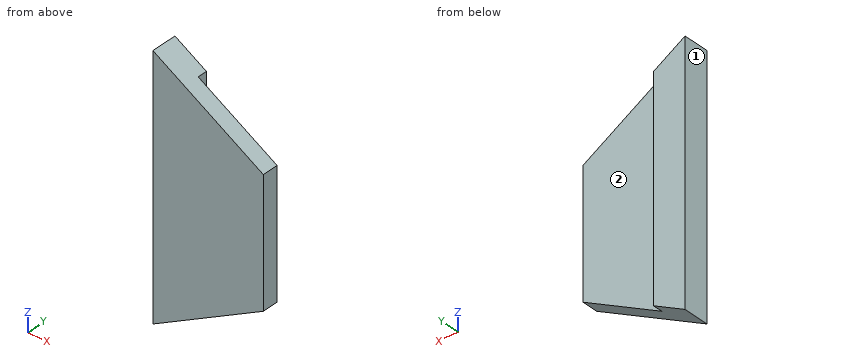
from build123d import *

# Parameters (mm, degrees)
SKETCH043_W      = 6
SKETCH043_H      = 16
EXTRUDE052_DEPTH = 1.6
EXTRUDE_DEPTH    = 1.6


with BuildPart() as extrude052:
    # Sketch043 → Extrude052 (new body)
    with BuildSketch(Plane.XZ.offset(-4.3)):
        with Locations((35, 12)):
            Rectangle(SKETCH043_W, SKETCH043_H)
    extrude(amount=EXTRUDE052_DEPTH)


with BuildPart() as body005:
    # Sketch → Extrude (new body)
    with BuildSketch(Plane.XZ.offset(-5.3)):
        Polygon((37, 16), (37, 8), (30, 4), (30, 20), align=None)
    extrude(amount=EXTRUDE_DEPTH)

    # Cut028: cut Extrude052
    add(extrude052.part, mode=Mode.SUBTRACT)


with BuildPart() as switch_protector001:
    # Part__Mirroring005: instance of Body005
    add(body005.part.mirror(Plane(origin=(0, 0, 0), x_dir=(1, 0, 0), z_dir=(0, 1, 0))))


solid = switch_protector001.part
Design review of the part built by this model. Coordinates are the model's own, in mm. Face numbers are marked on the shaded views. A direction names the side the tool comes from. Coordinates: 2 decimals unless noted, no trailing zeros. Order: outer loops, then holes, each group sorted by start corner. A loop starts at its lowest first (then second) coordinate and runs counter-clockwise, first axis right, second up. Notation, with made-up numbers: (7.25, 6.5) - (20.25, 6.5) arc R10 ccw to (20.25, 24.5) - close; hole circle Ø4 at (12, 38.25). An arc over 180 degrees is marked (long way). Put each result on its own line as item: value.
1) Wall thickness on L1, parallel to X at y = -4.05, z = 18.5; L2, parallel to Y at x = 34.25, z = 7.5; L3, parallel to X at y = -4.5, z = 17: over which ranges is each line inside the solid? List them lowest first. Write a range as from..to.
Response values:
L1: x = 30..32
L2: y = -5.3..-4.3
L3: x = 30..35.25
2) Insertion check: P1, Ø1.5, axis at x = 35, z = 11, coming from the +Y side; P2, Ø0.5, axis at y = -4, z = 13.5, coming from the +X side. Each pin has a flat end and moves straight along its axis. Give the tip position at first contact, or say it passes through.
Response values:
P1: stops at y = -4.3
P2: stops at x = 32
3) Tool access review of the marked faces 1 and 2: name each direction out of +Z, -Z, +X, -X, +Y, -Y from which nothing blocks a thin tool from reaching the whole face with its end or side.
Response values:
face 1: +Z, -Z, -X, +Y, -Y
face 2: +Z, -Z, +X, +Y
4) Take a section at C-C, the plane y = -4.5. Give the boundary of the cut face in (x, z).
Response values:
outline: (30, 4) - (37, 8) - (37, 16) - (30, 20) - close
5) Take a section at A-A, the plane z = 13.25. Give the boundary of the cut face in (x, y), and give its area (3 significant figures).
Response values:
outline: (30, -5.3) - (37, -5.3) - (37, -4.3) - (32, -4.3) - (32, -3.7) - (30, -3.7) - close
area: 8.20 mm²
6) Take a section at D-D, the plane z = 17. Give the boundary of the cut face in (x, y).
Response values:
outline: (30, -5.3) - (35.25, -5.3) - (35.25, -4.3) - (32, -4.3) - (32, -3.7) - (30, -3.7) - close
7) Take a section at B-B, the plane x = 33.5. Give the boundary of the cut face in (y, z), and give its area (3 significant figures).
Response values:
outline: (-5.3, 6) - (-4.3, 6) - (-4.3, 18) - (-5.3, 18) - close
area: 12.0 mm²
